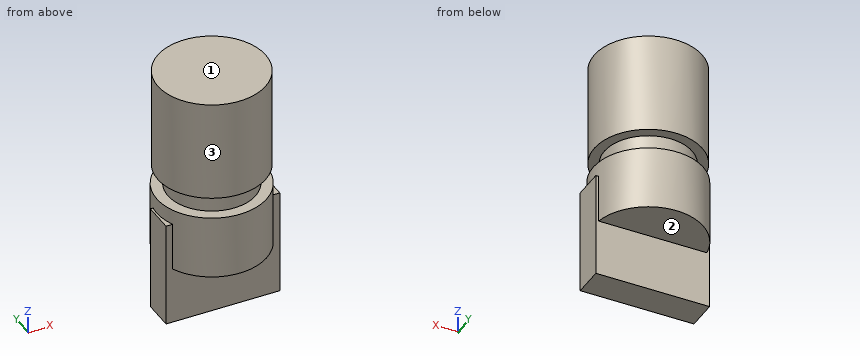
from build123d import *

# Parameters (mm, degrees)
SKETCH3_R           = 3
BOSS_EXTRUDE1_DEPTH = 5.63
SKETCH8_R           = 2.44
BOSS_EXTRUDE2_DEPTH = 1.16
SKETCH9_R           = 3.055
BOSS_EXTRUDE3_DEPTH = 3.55
BOSS_EXTRUDE4_START = 0.485
SKETCH15_W          = 6.34
SKETCH15_H          = 5.9
BOSS_EXTRUDE4_DEPTH = 1.7


with BuildPart() as part:
    # Sketch3 → Boss-Extrude1 (new body)
    with BuildSketch(Plane.XY):
        with Locations((-7.67170946, 4.798899109)):
            Circle(SKETCH3_R)
    extrude(amount=BOSS_EXTRUDE1_DEPTH)

    # Sketch8 → Boss-Extrude2 (add)
    with BuildSketch(Plane(origin=(0, 0, 0), x_dir=(-1, 0, 0), z_dir=(0, 0, -1))):
        with Locations(Location((7.67170946, 4.798899109, 0), (0, 0, 180))):
            Circle(SKETCH8_R)
    extrude(amount=BOSS_EXTRUDE2_DEPTH)

    # Sketch9 → Boss-Extrude3 (add)
    with BuildSketch(Plane(origin=(0, 0, -1.16), x_dir=(-1, 0, 0), z_dir=(0, 0, -1))):
        with Locations((7.67170946, 4.798899109)):
            Circle(SKETCH9_R)
    extrude(amount=BOSS_EXTRUDE3_DEPTH)

    # Sketch15 → Boss-Extrude4 (add)
    with BuildSketch(Plane(origin=(0, 4.798899109, 0), x_dir=(1, 0, 0), z_dir=(0, 1, 0)).offset(BOSS_EXTRUDE4_START)):
        with Locations((-7.67170946, 4.96)):
            Rectangle(SKETCH15_W, SKETCH15_H)
    extrude(amount=-BOSS_EXTRUDE4_DEPTH)


solid = part.part
Source: CAD feature listing. Evaluate the final solid. Frame: model axes, mm. Face numbers are marked on the shaded views. A direction names the side the tool comes from. Give positions to 0.01 mm unless a question says otherwise; leave off trailing zeros. Write each loop counter-clockwise with the first axis right and the second up, starting at its lowest first coordinate (ties: lowest second). Pieces come first, ordered by that corner, then holes. Notation, with made-up numbers: (52, 79) -> (76, 79) arc R23 cw to (76, 118) -> close; hole circle Ø7 at (49, 37.25). An arc over 180 degrees is marked (long way). Return JSON: item names as keys, results as strings. Group by question number.
1. Pin query (flat end, axial travel): pin 1 Ø1.3 at (x, y) = (-9, 6) entering from -Z; pin 2 Ø1.8 at (x, z) = (-8, -6) entering from +Y; pin 3 Ø3 at (y, z) = (7, -4) entering from +X. Return the tip coordinate at first contact, or that it passes through.
2. Section B-B, the plane x = -6.25. Output: boundary loops of the cut face in (y, z).
3. Access query for the marked faces 1, 2 and 3. Directions: +Z, -Z, +X, -X, +Y, -Y. A direction counts if a zero-diameter tool reaches every point of the face in a straight line with its end or side. Return the directions, or none.
4. Section D-D, the plane x = -9.75. Output: boundary loops of the cut face in (y, z).
5. Section C-C, the plane y = 2.5. Output: boundary loops of the cut face in (x, z), then the cut area to 3 significant figures.
6. Material intervals for line 1 (Z direction, x = -6.5, y = 2.5); line 2 (Z direction, x = -8.25, y = 5.5); line 3 (Y direction, x = -5.5, z = -7), sorted ascending. Write a range as from..to.
7. Section A-A, the plane z = -2.25. Output: boundary loops of the cut face in (x, y) (3 decimals), then the cut area to 3 significant figures.
Determined:
{
 "1": {"pin 1": "stops at z = -4.71", "pin 2": "stops at y = 5.28", "pin 3": "stops at x = -4.7"},
 "2": {"outline": "(2.09, -4.71) -> (3.58, -4.71) -> (3.58, -7.91) -> (5.28, -7.91) -> (5.28, -4.71) -> (7.5, -4.71) -> (7.5, -1.16) -> (6.78, -1.16) -> (6.78, 0) -> (7.44, 0) -> (7.44, 5.63) -> (2.16, 5.63) -> (2.16, 0) -> (2.82, 0) -> (2.82, -1.16) -> (2.09, -1.16) -> close"},
 "3": {"face 1": "+Z, +X, -X, +Y, -Y", "face 2": "-Z, +X, -X, +Y", "face 3": "+Z"},
 "4": {"outline": "(2.56, -4.71) -> (3.58, -4.71) -> (3.58, -7.91) -> (5.28, -7.91) -> (5.28, -4.71) -> (7.04, -4.71) -> (7.04, -1.16) -> (6.08, -1.16) -> (6.08, 0) -> (6.96, 0) -> (6.96, 5.63) -> (2.64, 5.63) -> (2.64, 0) -> (3.52, 0) -> (3.52, -1.16) -> (2.56, -1.16) -> close"},
 "5": {"outline": "(-9.68, -4.71) -> (-5.66, -4.71) -> (-5.66, -1.16) -> (-6.85, -1.16) -> (-6.85, 0) -> (-5.74, 0) -> (-5.74, 5.63) -> (-9.6, 5.63) -> (-9.6, 0) -> (-8.49, 0) -> (-8.49, -1.16) -> (-9.68, -1.16) -> close", "area": "37.9 mm2"},
 "6": {"line 1": "z = -4.71..-1.16, 0..5.63", "line 2": "z = -4.71..5.63", "line 3": "y = 3.58..5.28"},
 "7": {"outline": "(-10.842, 3.584) -> (-10.475, 3.584) arc R3.055 ccw to (-4.869, 3.584) -> (-4.502, 3.584) -> (-4.502, 5.284) -> (-4.655, 5.284) arc R3.055 ccw to (-10.688, 5.284) -> (-10.842, 5.284) -> close", "area": "29.9 mm2"}
}
